```python
from build123d import *

# Parameters (mm, degrees)
SIDE_W                               = 35.95
SIDE_H                               = 6
AUFSATZ_LINEAR_AUSTRAGEN1_DEPTH      = 10.85
AUFSATZ_LINEAR_AUSTRAGEN1_DEPTH_BACK = 10.85
SKIZZE5_R                            = 1.25
SCHNITT_LINEAR_AUSTRAGEN1_DEPTH      = 11.85
SCHNITT_LINEAR_AUSTRAGEN1_DEPTH_BACK = 11.85


with BuildPart() as part:
    # Side → Aufsatz-Linear austragen1 (new body, two sides)
    with BuildSketch(Plane.XY) as aufsatz_linear_austragen1_sk:
        with Locations((5.375, 567)):
            Rectangle(SIDE_W, SIDE_H)
    extrude(amount=AUFSATZ_LINEAR_AUSTRAGEN1_DEPTH)
    extrude(aufsatz_linear_austragen1_sk.sketch, amount=-AUFSATZ_LINEAR_AUSTRAGEN1_DEPTH_BACK)

    # Skizze5 → Schnitt-Linear austragen1 (cut, two sides)
    with BuildSketch(Plane.XY) as schnitt_linear_austragen1_sk:
        with Locations((-8, 566.953897676)):
            Circle(SKIZZE5_R)
        with Locations((19.35, 566.953897676)):
            Circle(SKIZZE5_R)
    extrude(amount=SCHNITT_LINEAR_AUSTRAGEN1_DEPTH, mode=Mode.SUBTRACT)
    extrude(schnitt_linear_austragen1_sk.sketch, amount=-SCHNITT_LINEAR_AUSTRAGEN1_DEPTH_BACK, mode=Mode.SUBTRACT)


solid = part.part
```
Here's how the part is built. I have some questions about the finished solid (model axes, mm). Give positions to 0.01 mm unless a question says otherwise; leave off trailing zeros. Order: outer loops, then holes, each group sorted by start corner. A loop starts at its lowest first (then second) coordinate and runs counter-clockwise, first axis right, second up. Notation, with made-up numbers: (88.5, -18) - (136.5, -18) arc R18 ccw to (136.5, 9) - close; hole circle Ø10 at (-9.5, -9). An arc over 180 degrees is marked (long way). Answer as a JSON object with one key per item and string values. Group by question number.
Item 1: If we section it at A-A on x = 19.35: Please give me the cut outline in (y, z).
Item 2: Please list where these lines run through material, in increasing order: probe 1 along X at (y, z) = (567.05, 7.5); probe 2 along Y at (x, z) = (-8, 2.25); probe 3 along X at (y, z) = (567.65, 0.5).
Item 3: If we mould it in two halves opening along X, with no side actions, what happens to faces 1 (the flat face through (23.35, 567, 0)), 2 (the flat face through (-12.6, 567, 0)), 3 (the cylindrical face through (-8.163, 568.193, 0.152))? For each: pulls with the +X half, pulls with the -X half, needs draft (parallel to the pull), parting line crosses it, or undercut.
Item 4: If we section it at B-B on y = 567.6: Please give me the cut outline in (x, z), and give its area (3 significant figures).
Item 5: If we section it at C-C on z = -6.25: Please give me the cut outline in (x, y), and give its area (3 significant figures).
Result set:
{
 "1": {"outline": "(564, -10.85) - (565.7, -10.85) - (565.7, 10.85) - (564, 10.85) - close; (568.2, -10.85) - (570, -10.85) - (570, 10.85) - (568.2, 10.85) - close"},
 "2": {"probe 1": "-12.6 to -9.25, -6.75 to 18.1, 20.6 to 23.35", "probe 2": "564 to 565.7, 568.2 to 570", "probe 3": "-12.6 to -9.04, -6.96 to 18.31, 20.39 to 23.35"},
 "3": {"face 1": "pulls with the +X half", "face 2": "pulls with the -X half", "face 3": "undercut"},
 "4": {"outline": "(-12.6, -10.85) - (-9.07, -10.85) - (-9.07, 10.85) - (-12.6, 10.85) - close; (-6.93, -10.85) - (18.28, -10.85) - (18.28, 10.85) - (-6.93, 10.85) - close; (20.42, -10.85) - (23.35, -10.85) - (23.35, 10.85) - (20.42, 10.85) - close", "area": "687 mm²"},
 "5": {"outline": "(-12.6, 564) - (23.35, 564) - (23.35, 570) - (-12.6, 570) - close; hole circle Ø2.5 at (-8, 566.95); hole circle Ø2.5 at (19.35, 566.95)", "area": "206 mm²"}
}
